from build123d import *

# Parameters (mm, degrees)
FILLET1_R          = 0.3
CUT_EXTRUDE1_DEPTH = 2.4
CHAMFER1_SIZE      = 0.2


with BuildPart() as part:
    # Sketch1 → Revolve1 (revolve)
    with BuildSketch(Plane.XY):
        Polygon((0, 3.5), (-4.5, 3.5), (-4.5, 0), (-2.5, 0), (-2.5, -25), (-2, -25), (-2, -33), (0, -33), align=None)
    revolve(axis=Axis((0, 3.5, 0), (0, -1, 0)))

    # Fillet1
    fillet1_edges = [part.edges().sort_by_distance(p)[0] for p in [
        (4.5, 0, 0),
        (4.5, 3.5, 0),
    ]]
    fillet(fillet1_edges, radius=FILLET1_R)

    # Sketch2 → Cut-Extrude1 (cut)
    with BuildSketch(Plane(origin=(0, 3.5, 0), x_dir=(1, 0, 0), z_dir=(0, 1, 0))):
        Polygon((1.5, 0.866025404), (0, 1.732050808), (-1.5, 0.866025404), (-1.5, -0.866025404), (0, -1.732050808), (1.5, -0.866025404), align=None)
    extrude(amount=-CUT_EXTRUDE1_DEPTH, mode=Mode.SUBTRACT)

    # Chamfer1
    chamfer1_edges = [part.edges().sort_by_distance(p)[0] for p in [
        (2.5, -25, 0),
    ]]
    chamfer(chamfer1_edges, length=CHAMFER1_SIZE)


solid = part.part
Could you check a few things on this model? Use its own coordinates, in mm. A direction names the side the tool comes from. Give positions to 0.01 mm unless a question says otherwise; leave off trailing zeros. Order: outer loops, then holes, each group sorted by start corner. A loop starts at its lowest first (then second) coordinate and runs counter-clockwise, first axis right, second up.
1. Suppose I cut it at A-A (z = 0). List the corners of the cut face in (x, y) for me.
2. We'd pull the mould along Z, two halves only. Please class faces 1 (the cylindrical face through (0.54, -12.57, 2.44)), 2 (the flat face through (2, 3.5, 0)), 3 (the flat face through (0.74, 2.317, 1.305)): pulls with the +Z half, pulls with the -Z half, needs draft (parallel to the pull), parting line crosses it, or undercut.
3. Suppose I cut it at B-B (y = -13.5). List the corners of the cut face in (x, z) for me, plus the area to 3 significant figures.
4. Will these pins go through, and if not, where does the flat tip stop? P1, Ø2, axis at y = -28.5, z = -2, coming from the +X side; P2, Ø3, axis at x = 2, y = -1, coming from the -Z side; P3, Ø2, axis at x = -1.5, z = -3, coming from the -Y side.
5. For faces 4 (the cylindrical face through (0.59, 1.73, -4.46)), 5 (the cylindrical face through (0, -29, 2)), 6 (the flat face through (-0.76, 2.317, 1.293)), which set-ups out of +Z, -Z, +X, -X, +Y, -Y let a thin tool reach every point of the face, with its end or its side?
6. I need wall thicknesses on L1, parallel to Z at x = -1.5, y = -18; L2, parallel to Y at x = -2, z = -3.75; L3, parallel to X at y = -6.5, z = 0. Which ranges of each line are inside material? Lowest first, please.
Solved:
1. outline: (-4.5, 0.3) arc R0.3 ccw to (-4.2, 0) - (-2.5, 0) - (-2.5, -24.8) - (-2.3, -25) - (-2, -25) - (-2, -33) - (2, -33) - (2, -25) - (2.3, -25) - (2.5, -24.8) - (2.5, 0) - (4.2, 0) arc R0.3 ccw to (4.5, 0.3) - (4.5, 3.2) arc R0.3 ccw to (4.2, 3.5) - (1.5, 3.5) - (1.5, 1.1) - (-1.5, 1.1) - (-1.5, 3.5) - (-4.2, 3.5) arc R0.3 ccw to (-4.5, 3.2) - close
2. face 1: parting line crosses it
2. face 2: needs draft
2. face 3: undercut
3. outline: circle Ø5 at (0, 0)
3. area: 19.6 mm2
4. P1: stops at x = 1.73
4. P2: stops at z = -4.35
4. P3: stops at y = -24.95
5. face 4: +Y, -Y
5. face 5: -Y
5. face 6: +Y
6. L1: z = -2 to 2
6. L2: y = 0 to 3.5
6. L3: x = -2.5 to 2.5
